Could you check a few things on this model? Use its own coordinates, in mm. A direction names the side the tool comes from. Coordinates: 2 decimals unless noted, no trailing zeros. Order: outer loops, then holes, each group sorted by start corner. A loop starts at its lowest first (then second) coordinate and runs counter-clockwise, first axis right, second up. Notation, with made-up numbers: (16, 59.5) - (47, 59.5) arc R15 cw to (47, 74.5) - close; hole circle Ø7 at (78, -19.5). An arc over 180 degrees is marked (long way). Answer as a JSON object with one key per item and string values. Group by question number.
(1) We'd pull the mould along Z, two halves only. Please class faces 1 (the flat face through (4, 19, 130.175)), 2 (the flat face through (-11, -16, 0)), 3 (the cylindrical face through (15.12, 11.59, 128.61)), 4 (the cylindrical face through (-18.897, -14.49, 62.611)): pulls with the +Z half, pulls with the -Z half, needs draft (parallel to the pull), parting line crosses it, or undercut.
(2) Imagine slicing it at C-C, the plane z = 84.5. Write out the boundary of the cut face in (x, y) (1 decimal).
(3) Imagine slicing it at D-D, the plane y = 20.5. Write out the boundary of the cut face in (x, z) (1 decimal), and give its area (3 significant figures).
(4) Which directions (+Z, -Z, +X, -X, +Y, -Y) give clear straight access to the entire face, cutting with the end or side of a thin tool? Please do faces 5 (the flat face through (-11, 16, 127)), 6 (the cylindrical face through (15.12, 11.59, -1.57)).
(5) Will these pins go through, and if not, where does the flat tip stop? P1, Ø10, axis at y = -20, z = 47.5, coming from the +X side; P2, Ø10, axis at y = 15, z = 29, coming from the +X side; P3, Ø12, axis at x = -12, y = 3, coming from the -Z side; P4, Ø6, axis at x = 13.5, z = 92, coming from the -Y side.
(6) Please list where these lines run through material, in increasing order: probe 1 along Z at (x, y) = (6.5, -20.5) (3 decimals); probe 2 along Y at (x, z) = (0, -2.4); probe 3 along Y at (x, z) = (12.5, 88).
from build123d import *

# Parameters (mm, degrees)
F0_R     = 25.4
F0_R_2   = 23.8125
F1_DEPTH = 127
F2_R     = 25.4
F3_DEPTH = 3.175
F4_R     = 25.4
F5_DEPTH = 3.175
F7_D     = 38.1


with BuildPart() as f1:
    # F0 (on Top) → F1 (new body)
    with BuildSketch(Plane.XY):
        Circle(F0_R)
        Circle(F0_R_2, mode=Mode.SUBTRACT)
    extrude(amount=F1_DEPTH)

    # F2 (on face) → F3 (join)
    with BuildSketch(Plane.XY.offset(127)):
        Circle(F2_R)
    extrude(amount=F3_DEPTH)

    # F4 (on face) → F5 (join)
    with BuildSketch(Plane(origin=(0, 0, 0), x_dir=(1, 0, 0), z_dir=(0, 0, -1))):
        Circle(F4_R)
    extrude(amount=F5_DEPTH)

    # F7 (through all)
    with Locations(Plane(origin=(0, 0, -3.175), x_dir=(1, 0, 0), z_dir=(0, 0, -1))):
        with Locations((0, 0)):
            Hole(F7_D / 2)


solid = f1.part
Result set:
{
 "1": {"face 1": "pulls with the +Z half", "face 2": "undercut", "face 3": "needs draft", "face 4": "undercut"},
 "2": {"outline": "circle Ø50.8 at (0, 0); hole circle Ø47.6 at (0, 0)"},
 "3": {"outline": "(-15, -3.2) - (15, -3.2) - (15, 130.2) - (-15, 130.2) - close; hole (-12.1, 0) - (12.1, 0) - (12.1, 127) - (-12.1, 127) - close", "area": "922 mm^2"},
 "4": {"face 5": "none", "face 6": "+Z, -Z"},
 "5": {"P1": "stops at x = 20.5", "P2": "stops at x = 23.35", "P3": "passes through", "P4": "stops at y = -23.13"},
 "6": {"probe 1": "z = -3.175 to 0, 127 to 130.175", "probe 2": "y = -25.4 to -19.05, 19.05 to 25.4", "probe 3": "y = -22.11 to -20.27, 20.27 to 22.11"}
}
